```python
from build123d import *

# Parameters (mm, degrees)
F0_W     = 150
F0_H     = 44
F1_DEPTH = 1600
F4_W     = 22
F4_H     = 120
F5_DEPTH = 44
F6_W     = 128
F6_H     = 120
F7_DEPTH = 22


# Not quite as in the source:
# - a pattern or mirror of a feature is missing from the dataset's text; its kind, count and spacing are read off the source's solid


with BuildPart() as f1:
    # F0 (on Front) → F1 (new body)
    with BuildSketch(Plane.XZ):
        with Locations((-75, 22)):
            Rectangle(F0_W, F0_H)
    extrude(amount=-F1_DEPTH)

    # F4 (on face) → F5 (cut, through all)
    with BuildSketch(Plane.XY.offset(44)):
        with Locations((-11, 1540)):
            Rectangle(F4_W, F4_H)
    f5 = extrude(amount=-F5_DEPTH, mode=Mode.SUBTRACT)

    # F5_copies: F5 across plane
    add(f5.mirror(Plane(origin=(0, 800, 0), x_dir=(0, 0, -1), z_dir=(0, -1, 0))), mode=Mode.SUBTRACT)

    # F6 (on face) → F7 (cut)
    with BuildSketch(Plane.XY.offset(44)):
        with Locations((-86, 1540)):
            Rectangle(F6_W, F6_H)
    f7 = extrude(amount=-F7_DEPTH, mode=Mode.SUBTRACT)

    # F7_copies: F7 across plane
    add(f7.mirror(Plane(origin=(0, 800, 0), x_dir=(0, 0, -1), z_dir=(0, -1, 0))), mode=Mode.SUBTRACT)


solid = f1.part
```
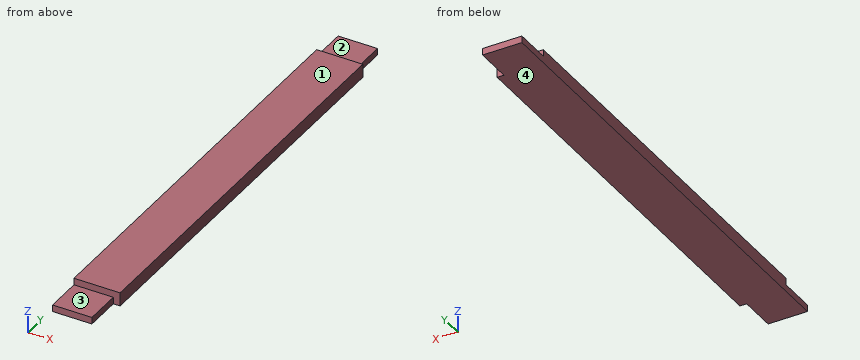
Build history of the part. All positions in model axes, mm. Face numbers are marked on the shaded views. A direction names the side the tool comes from. Coordinates: 2 decimals unless noted, no trailing zeros. Order: outer loops, then holes, each group sorted by start corner. A loop starts at its lowest first (then second) coordinate and runs counter-clockwise, first axis right, second up.
Item 1: Drill centre lines: L1, parallel to Y at x = -20, z = 24; L2, parallel to Z at x = -130.5, y = 92; L3, parallel to X at y = 102, z = 10. Where is each one in solid material? Low to high.
Filled in:
L1: y = 120 to 1480
L2: z = 0 to 22
L3: x = -150 to -22
Item 2: Drop flat-ended pins along their axis: pin 1 Ø17.5 at (y, z) = (52.5, 13.5) entering from +X; pin 2 Ø3 at (x, z) = (-124.5, 39) entering from -Y. Give the stop position or say it passes through.
Filled in:
pin 1: stops at x = -22
pin 2: stops at y = 120
Item 3: Saw through at B-B on x = -79.5. List the corners of the cut face in (y, z), then the cut area to 3 significant figures.
Filled in:
outline: (0, 0) - (1600, 0) - (1600, 22) - (1480, 22) - (1480, 44) - (120, 44) - (120, 22) - (0, 22) - close
area: 65,100 mm2
Item 4: Saw through at A-A on z = 10. List the corners of the cut face in (x, y).
Filled in:
outline: (-150, 0) - (-22, 0) - (-22, 120) - (0, 120) - (0, 1480) - (-22, 1480) - (-22, 1600) - (-150, 1600) - close
Item 5: Tool access for the marked faces 1 and 2: list every direction of +Z, -Z, +X, -X, +Y, -Y with a clear straight run to the whole face (end or side of a thin tool).
Filled in:
face 1: +Z, +X, -X, +Y, -Y
face 2: +Z, +X, -X, +Y
Item 6: Mould opens along Z. For the marked faces 3 and 4 say: released by +Z, released by -Z, zero draft, split by the parting line, or undercut.
Filled in:
face 3: released by +Z
face 4: released by -Z
